Model file for the job. Use its own axes, mm. Face numbers are marked on the shaded views. Round coordinates to 2 decimals unless told otherwise and drop trailing zeros. Order: outer loops, then holes, each group sorted by start corner. A loop starts at its lowest first (then second) coordinate and runs counter-clockwise, first axis right, second up. Notation, with made-up numbers: (69, 62.25) - (106, 62.25) arc R34 ccw to (106, 93.25) - close; hole circle Ø11 at (-38.5, 49). An arc over 180 degrees is marked (long way). Put each result on its own line as item: value. Start each with the question number.
Item 1: Probe probe 1 along Y at (x, z) = (-38, 7.5); probe 2 along X at (y, z) = (-662, 4.25); probe 3 along X at (y, z) = (-701, 4). List the from-to ranges inside material, lowest first.
Item 2: Saw through at C-C on y = -713. List the corners of the cut face in (x, z), plus the area to 3 significant figures.
Item 3: Saw through at A-A on y = -790. List the corners of the cut face in (x, z).
Item 4: Pin check, flat tips, straight feed: pin 1 Ø6 at (x, y) = (32, -746) entering from +Z; pin 2 Ø10.5 at (x, y) = (-26, -690) entering from +Z. Stop position of each tip, or through.
Item 5: Mould opens along X. For the marked faces 1 and 2 say: pulls with the +X half, pulls with the -X half, needs draft (parallel to the pull), parting line crosses it, or undercut.
Item 6: Saw through at B-B on z = 5.5. State how many separate pieces and enclosed holes the cut face has, plus the area to 3 significant figures.
Item 7: Saw through at D-D on y = -771. List the corners of the cut face in (x, z), plus the area to 3 significant figures.
```python
from build123d import *

# Parameters (mm, degrees)
PAD004_DEPTH    = 9.8
SKETCH080_R     = 37.95
PAD016_DEPTH    = 11.8
SKETCH081_R     = 5.5
SKETCH081_R_2   = 6.5
SKETCH081_R_3   = 8.5
SKETCH081_R_4   = 14
SKETCH081_R_5   = 16
POCKET007_DEPTH = 8
SKETCH082_R     = 1.5
SKETCH082_R_2   = 4
SKETCH082_R_3   = 2.4
SKETCH082_R_4   = 3
SKETCH082_R_5   = 6
SKETCH082_R_6   = 5
POCKET008_DEPTH = 11.801


with BuildPart() as part:
    # Sketch041 → Pad004 (new body)
    with BuildSketch(Plane.XY):
        with BuildLine():
            Line((-48, 145), (-48, 3))
            ThreePointArc((-48, 3), (-47.12132, 0.87868), (-45, 0))
            Line((-45, 0), (45, 0))
            ThreePointArc((45, 0), (47.12132, 0.87868), (48, 3))
            Line((48, 145), (48, 3))
            ThreePointArc((48, 145), (47.12132, 147.12132), (45, 148))
            Line((-45, 148), (45, 148))
            ThreePointArc((-45, 148), (-47.12132, 147.12132), (-48, 145))
        make_face()
    extrude(amount=PAD004_DEPTH)

    # Sketch080 (on Pad) → Pad016 (join)
    with BuildSketch(Plane.XY):
        with Locations((0, 100)):
            Circle(SKETCH080_R)
    extrude(amount=PAD016_DEPTH)

    # Sketch081 (on Face13 of Pad016) → Pocket007 (cut)
    with BuildSketch(Plane.XY.offset(11.8)):
        with Locations((-16.188435, 123.395236)):
            Circle(SKETCH081_R)
        with Locations((-25.430368, 110.334353)):
            Circle(SKETCH081_R_2)
        with Locations((-23.950087, 91.392105)):
            Circle(SKETCH081_R_3)
        with Locations((0, 80.05)):
            Circle(SKETCH081_R_4)
        with Locations((14.244595, 110.92218)):
            Circle(SKETCH081_R_5)
    extrude(amount=-POCKET007_DEPTH, mode=Mode.SUBTRACT)

    # Sketch082 (on Face13 of Pocket007) → Pocket008 (cut, through all)
    with BuildSketch(Plane.XY.offset(11.8)):
        with Locations((-38, 138)):
            Circle(SKETCH082_R)
        with Locations((38, 138)):
            Circle(SKETCH082_R)
        with Locations((14.244595, 110.92218)):
            Circle(SKETCH082_R_2)
        with Locations((3.044595, 110.92218)):
            Circle(SKETCH082_R_3)
        with Locations((-16.188435, 123.395236)):
            Circle(SKETCH082_R_4)
        with Locations((-25.430368, 110.334353)):
            Circle(SKETCH082_R_2)
        with Locations((-23.950087, 91.392105)):
            Circle(SKETCH082_R_5)
        with Locations((0, 80.05)):
            Circle(SKETCH082_R_6)
        with Locations((-38, 10)):
            Circle(SKETCH082_R)
        with Locations((38, 10)):
            Circle(SKETCH082_R)
    extrude(amount=-POCKET008_DEPTH, mode=Mode.SUBTRACT)


with BuildPart() as part_1:
    # Body002 placement: moved
    add(part.part.moved(Location((0, -800, 0))))


solid = part_1.part
```
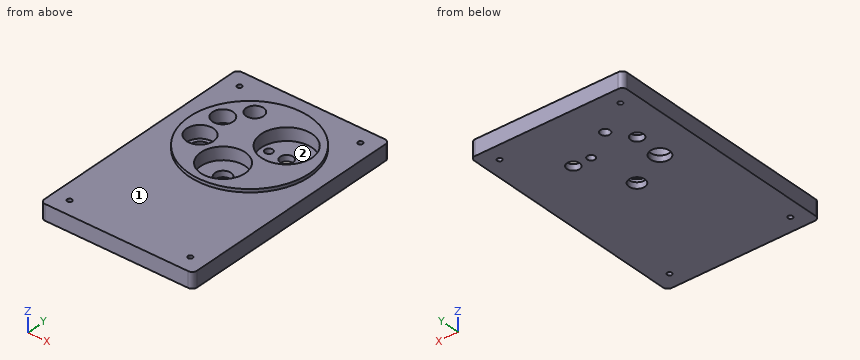
Results found:
1. probe 1: y = -800 to -791.5, -788.5 to -663.5, -660.5 to -652
1. probe 2: x = -48 to -39.5, -36.5 to 36.5, 39.5 to 48
1. probe 3: x = -48 to -27.74, -20.16 to 3.57, 24.92 to 48
2. outline: (-48, 0) - (-28.04, 0) - (-28.04, 3.8) - (-31.23, 3.8) - (-31.23, 11.8) - (-35.65, 11.8) - (-35.65, 9.8) - (-48, 9.8) - close; (-19.86, 0) - (48, 0) - (48, 9.8) - (35.65, 9.8) - (35.65, 11.8) - (12.15, 11.8) - (12.15, 3.8) - (-12.15, 3.8) - (-12.15, 11.8) - (-16.67, 11.8) - (-16.67, 3.8) - (-19.86, 3.8) - close
2. area: 741 mm²
3. outline: (-48, 0) - (-39.5, 0) - (-39.5, 9.8) - (-48, 9.8) - close; (-36.5, 0) - (36.5, 0) - (36.5, 9.8) - (-36.5, 9.8) - close; (39.5, 0) - (48, 0) - (48, 9.8) - (39.5, 9.8) - close
4. pin 1: stops at z = 9.8
4. pin 2: stops at z = 3.8
5. face 1: needs draft
5. face 2: undercut
6. separate pieces: 1
6. enclosed holes: 9
6. area: 12,300 mm²
7. outline: (-48, 0) - (48, 0) - (48, 9.8) - (-48, 9.8) - close
7. area: 941 mm²
